Part model, mm, in its own coordinate system. A direction names the side the tool comes from. Round coordinates to 2 decimals unless told otherwise and drop trailing zeros. Write each loop counter-clockwise with the first axis right and the second up, starting at its lowest first coordinate (ties: lowest second). Pieces come first, ordered by that corner, then holes.
```python
from build123d import *

# Parameters (mm, degrees)
F1_DEPTH = 25
F2_W     = 10
F2_H     = 284.1381265149
F3_DEPTH = 10


with BuildPart() as f1:
    # F0 (on Front) → F1 (new body)
    with BuildSketch(Plane.XZ):
        Polygon((-175, 0), (175, 0), (200, 150), (110, 150), (110, 125), (100, 125), (100, 150), (80, 150), (80, 125), (70, 125), (70, 150), (50, 150), (50, 125), (40, 125), (40, 150), (20, 150), (20, 125), (10, 125), (10, 150), (-10, 150), (-10, 125), (-20, 125), (-20, 150), (-40, 150), (-40, 125), (-50, 125), (-50, 150), (-70, 150), (-70, 125), (-80, 125), (-80, 150), (-100, 150), (-100, 125), (-110, 125), (-110, 150), (-200, 150), align=None)
        Polygon((110, -150), (150, -150), (175, 0), (-175, 0), (-150, -150), (-110, -150), (-110, -125), (-100, -125), (-100, -150), (-80, -150), (-80, -125), (-70, -125), (-70, -150), (-50, -150), (-50, -125), (-40, -125), (-40, -150), (-20, -150), (-20, -125), (-10, -125), (-10, -150), (10, -150), (10, -125), (20, -125), (20, -150), (40, -150), (40, -125), (50, -125), (50, -150), (70, -150), (70, -125), (80, -125), (80, -150), (100, -150), (100, -125), (110, -125), align=None)
    extrude(amount=F1_DEPTH)

    # F2 (on face) → F3 (cut)
    with BuildSketch(Plane(origin=(170.2702702703, 0, -28.3783783784), x_dir=(0, 1, 0), z_dir=(0.9863939238, 0, -0.1643989873))):
        with Locations((-5, 28.7698227784)):
            Rectangle(F2_W, F2_H)
    extrude(amount=-F3_DEPTH, mode=Mode.SUBTRACT)


solid = f1.part
```
Q1. Mould opens along X. For faces 1 (the flat face through (146.781, -5.07, -139.326)), 2 (the flat face through (-100, -12, -137)), 3 (the flat face through (-10, -12, 138)), 4 (the flat face through (-30, -12, 150)) say: +X half, -X half, draft (parallel to the pull), parting line (faces both ways), or undercut.
Values follow:
face 1: +X half
face 2: undercut
face 3: undercut
face 4: draft
Q2. Drop flat-ended pins along their axis: pin 1 (12 mm diameter, centred on y = -3, z = -75, fed in from +X); pin 2 (12.5 mm diameter, centred on y = -7, z = -133.5, fed in from -X); pin 3 (7.5 mm diameter, centred on y = -7.5, z = 143.5, fed in from -X). Give the stop position or say it passes through.
Values follow:
pin 1: stops at x = 153.36
pin 2: stops at x = -153.79
pin 3: stops at x = -199.54
Q3. Cut at B-B on x = -160.5. Write the cut outline in (y, z), plus the area to 4 significant figures.
Values follow:
outline: (-25, -87) - (0, -87) - (0, 150) - (-25, 150) - close
area: 5,925 mm2
Q4. Which spindle directions (+Z, -Z, +X, -X, +Y, -Y) get a long thin tool onto all of the face, cutting with end or side? Do faces 5 (the flat face through (-154, -12, 150)), 6 (the flat face through (80, -12, 138)), 7 (the flat face through (50, -12, -137)). Say none if no direction does.
Values follow:
face 5: +Z, +X, -X, +Y, -Y
face 6: +Z, +Y, -Y
face 7: -Z, +Y, -Y
Q5. Wall check: L1, parallel to Z at x = -43, y = -2.5; L2, parallel to X at y = -20.25, z = 99.5; L3, parallel to X at y = -4.5, z = -104. Give the ranges that are in metal, low to high.
Values follow:
L1: z = -125 to 125
L2: x = -191.58 to 191.58
L3: x = -157.67 to 147.53
Q6. Cut at A-A on z = 50. Write the cut outline in (x, y).
Values follow:
outline: (-183.33, -25) - (183.33, -25) - (183.33, -10) - (173.2, -10) - (173.2, 0) - (-183.33, 0) - close
Q7. Cut at C-C on z = -65. Write the cut outline in (x, y), plus the area to 3 significant figures.
Values follow:
outline: (-164.17, -25) - (164.17, -25) - (164.17, -10) - (154.03, -10) - (154.03, 0) - (-164.17, 0) - close
area: 8,110 mm2
